Design review of the part built by this model. Coordinates are the model's own, in mm. A direction names the side the tool comes from. Coordinates: 2 decimals unless noted, no trailing zeros. Order: outer loops, then holes, each group sorted by start corner. A loop starts at its lowest first (then second) coordinate and runs counter-clockwise, first axis right, second up. Notation, with made-up numbers: (82, 81) - (105, 81) arc R27 cw to (105, 115) - close; hole circle Ø8 at (13, -8.5). An arc over 180 degrees is marked (long way). Write each question's results on one line, items separated by ' | '. Start each with the question number.
```python
from build123d import *

# Parameters (mm, degrees)
SKETCH1_R           = 6
BOSS_EXTRUDE2_DEPTH = 3
SKETCH4_R           = 6
BOSS_EXTRUDE3_DEPTH = 6.5
SKETCH5_R           = 1.1
CUT_EXTRUDE2_DEPTH  = 6.5
SKETCH6_R           = 1.5
SKETCH6_R_2         = 1.3
CUT_EXTRUDE3_DEPTH  = 0.1
SKETCH7_R           = 0.3
BOSS_EXTRUDE4_DEPTH = 2


with BuildPart() as part:
    # Sketch1 → Boss-Extrude2 (new body)
    with BuildSketch(Plane.XY):
        Circle(SKETCH1_R)
    extrude(amount=BOSS_EXTRUDE2_DEPTH)

    # Sketch4 → Boss-Extrude3 (add)
    with BuildSketch(Plane.XY.offset(3)):
        Circle(SKETCH4_R)
    extrude(amount=BOSS_EXTRUDE3_DEPTH)

    # Sketch5 → Cut-Extrude2 (cut)
    with BuildSketch(Plane.XY.offset(9.5)):
        Circle(SKETCH5_R)
    extrude(amount=-CUT_EXTRUDE2_DEPTH, mode=Mode.SUBTRACT)

    # Sketch6 → Cut-Extrude3 (cut)
    # profile 1 of 2: a face of its own
    with BuildSketch(Plane.XY.offset(9.5)):
        with Locations((0, 3.55)):
            Circle(SKETCH6_R)
        with Locations((0, 3.55)):
            Circle(SKETCH6_R_2, mode=Mode.SUBTRACT)
    # profile 2 of 2: a face of its own
    with BuildSketch(Plane.XY.offset(9.5)):
        Polygon((-0.15, 2.75), (0.15, 2.75), (0.15, 3.4), (0.8, 3.4), (0.8, 3.55), (0.8, 3.7), (0.15, 3.7), (0.15, 4.35), (-0.15, 4.35), (-0.15, 3.7), (-0.8, 3.7), (-0.8, 3.4), (-0.15, 3.4), align=None)
    extrude(amount=-CUT_EXTRUDE3_DEPTH, mode=Mode.SUBTRACT)

    # Sketch7 → Boss-Extrude4 (add)
    with BuildSketch(Plane(origin=(0, 0, 0), x_dir=(-1, 0, 0), z_dir=(0, 0, -1))):
        with Locations(Location((0, 3.8, 0), (0, 0, 180))):
            Circle(SKETCH7_R)
        with Locations(Location((0, -3.8, 0), (0, 0, 180))):
            Circle(SKETCH7_R)
    extrude(amount=BOSS_EXTRUDE4_DEPTH)


solid = part.part
```
(1) To check wall thickness, follow line 1 along Y through (x, z) = (0, 9.45); line 2 along Y through (x, z) = (0, 7); line 3 along Z through (x, y) = (-1.5, -2). State the ranges of each line that lie inside material, in increasing order. Write a range as [from, to].
(2) Take a section at D-D (y = -3.8). State the section outline as (x, z) points, plus the area to 3 significant figures.
(3) Mouldability with a two-part tool opening along Y and no side actions: class faces 3 (the face through (0, 0, 3)), 4 (the face through (-6, 0, 5)), 5 (the face through (-0.31, 3.86, 9.5)) as +Y half, -Y half, draft (parallel to the pull), parting line (faces both ways), or undercut.
(4) Take a section at C-C (x = -4.25). State the section outline as (y, z) points.
(5) Clearance check with flat-ended pins moving along their axes: pin 1 (1.8 mm diameter, centred on x = 0, y = 0, fed in from +Z); pin 2 (3 mm diameter, centred on x = -2.5, y = -1, fed in from -Z); pin 3 (6 mm diameter, centred on y = -4.5, z = 1, fed in from -X). State where each tip first meets the part, or that it passes through.
(6) Take a section at A-A (y = 0). State the section outline as (x, z) points.
(7) Tool access review of faces 1 (the face through (1.05, 0.33, 6.3)), 2 (the face through (-0.08, -1.25, 9.5)): name each direction out of +Z, -Z, +X, -X, +Y, -Y from which nothing blocks a thin tool from reaching the whole face with its end or side.
(8) Take a section at B-B (z = 8.5). State the section outline as (x, y) points, plus the area to 3 significant figures.
Worked out:
1) line 1: [-6, -1.1], [1.1, 2.05], [2.25, 2.75], [4.35, 4.85], [5.05, 6] | line 2: [-6, -1.1], [1.1, 6] | line 3: [0, 9.5]
2) outline: (-4.64, 0) - (-0.3, 0) - (-0.3, -2) - (0.3, -2) - (0.3, 0) - (4.64, 0) - (4.64, 9.5) - (-4.64, 9.5) - close | area: 89.4 mm^2
3) face 3: undercut | face 4: parting line | face 5: draft
4) outline: (-4.24, 0) - (4.24, 0) - (4.24, 9.5) - (-4.24, 9.5) - close
5) pin 1: z = 3 | pin 2: z = 0 | pin 3: x = -5.81
6) outline: (-6, 0) - (6, 0) - (6, 9.5) - (1.1, 9.5) - (1.1, 3) - (-1.1, 3) - (-1.1, 9.5) - (-6, 9.5) - close
7) face 1: +Z | face 2: +Z, +X, -X, +Y, -Y
8) outline: circle Ø12 at (0, 0); hole circle Ø2.2 at (0, 0) | area: 109 mm^2
